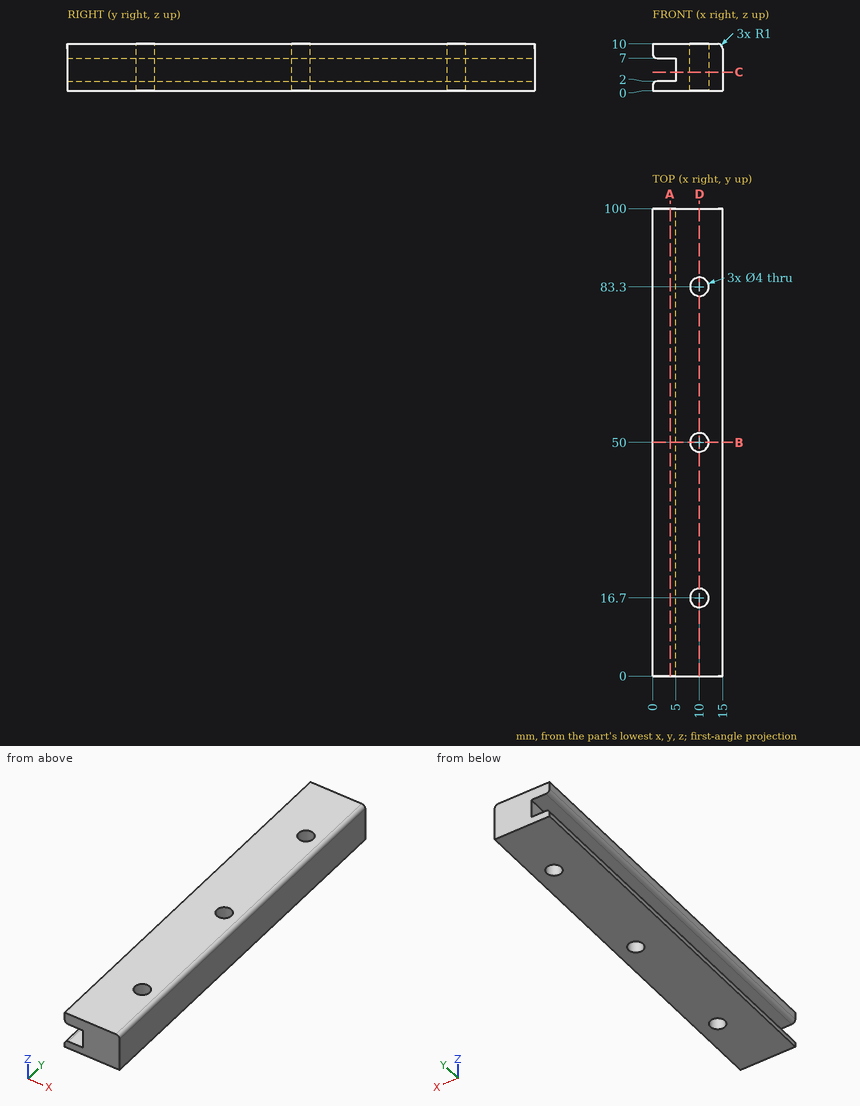
Here's the drawing with two shaded views (mm, measured from the low corner). I have some questions. Round coordinates to 2 decimals unless told otherwise and drop trailing zeros. Loops run counter-clockwise (first coordinate to the right, second up) from the corner with the lowest first, then second, coordinate; pieces in that order, holes last.
1. Suppose I cut it at A-A, the plane x = 3.75. Please give me the cut outline in (y, z).
Answers:
outline: (0, 0) - (100, 0) - (100, 2) - (0, 2) - close; (0, 7) - (100, 7) - (100, 10) - (0, 10) - close
2. Will these pins go through, and if not, where does the flat tip stop? pin 1 (1.5 mm diameter, centred on x = 9.5, y = 25.5, fed in from -Z); pin 2 (3.5 mm diameter, centred on x = 10, y = 50, fed in from -Z); pin 3 (1.5 mm diameter, centred on y = 74, z = 6.5, fed in from -X).
Answers:
pin 1: stops at z = 0
pin 2: passes through
pin 3: stops at x = 0.34
3. If I drill on probe 1 along Y at (x, z) = (10, 3.25); probe 2 along Z at (x, y) = (4.5, 84); probe 3 along X at (y, z) = (74, 6), over which ranges is the centre line in solid material (lowest first)?
Answers:
probe 1: y = 0 to 14.7, 18.7 to 48, 52 to 81.3, 85.3 to 100
probe 2: z = 0 to 2, 7 to 10
probe 3: x = 5 to 15
4. Suppose I cut it at D-D, the plane x = 10. Please give me the cut outline in (y, z), and give its area (3 significant figures).
Answers:
outline: (0, 0) - (14.7, 0) - (14.7, 10) - (0, 10) - close; (18.7, 0) - (48, 0) - (48, 10) - (18.7, 10) - close; (52, 0) - (81.3, 0) - (81.3, 10) - (52, 10) - close; (85.3, 0) - (100, 0) - (100, 10) - (85.3, 10) - close
area: 880 mm2
5. Suppose I cut it at B-B, the plane y = 50. Please give me the cut outline in (x, z), and give its area (3 significant figures).
Answers:
outline: (0, 0) - (8, 0) - (8, 10) - (0, 10) - (0, 8) arc R1 ccw to (1, 7) - (5, 7) - (5, 2) - (1, 2) arc R1 ccw to (0, 1) - close; (12, 0) - (15, 0) - (15, 9) arc R1 ccw to (14, 10) - (12, 10) - close
area: 84.4 mm2
6. Suppose I cut it at C-C, the plane z = 4. Please give me the cut outline in (x, y).
Answers:
outline: (5, 0) - (15, 0) - (15, 100) - (5, 100) - close; hole circle Ø4 at (10, 16.7); hole circle Ø4 at (10, 50); hole circle Ø4 at (10, 83.3)
